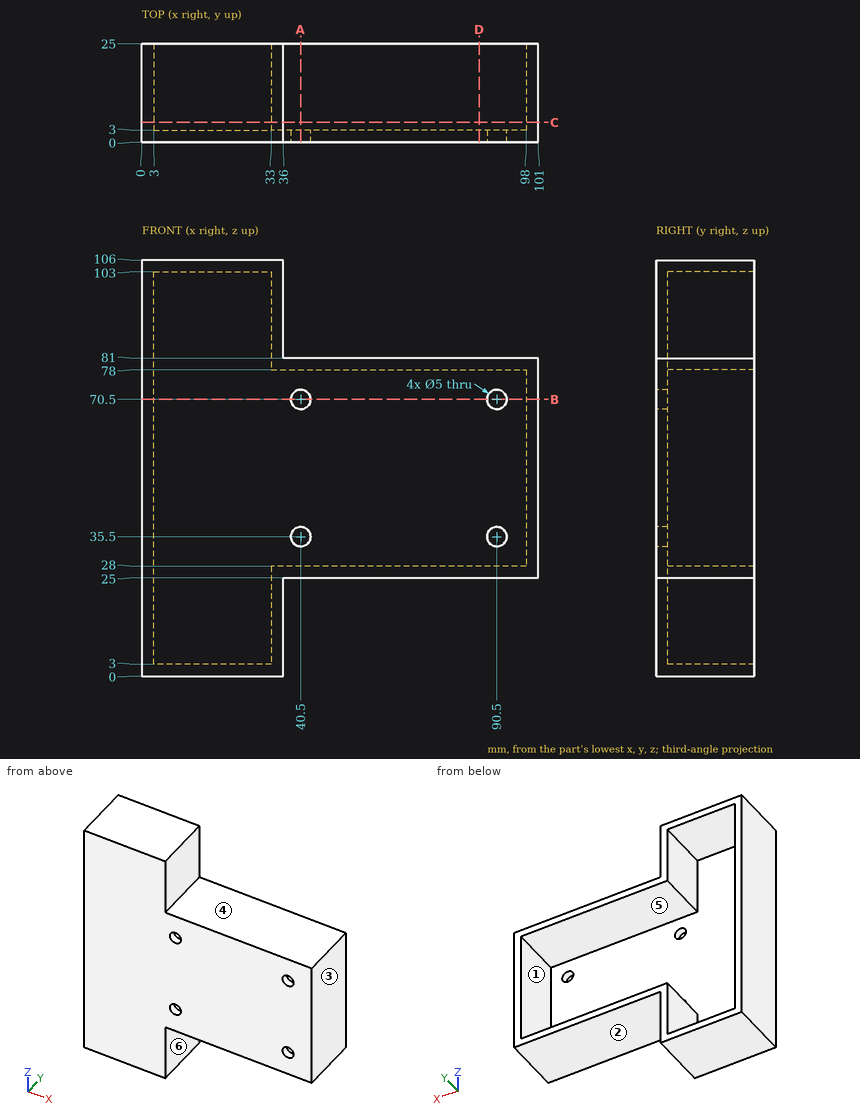
Part print with two shaded views. Sizes in mm from the minimum x, y, z corner. A direction names the side the tool comes from. Give positions to 0.01 mm unless a question says otherwise; leave off trailing zeros. Order: outer loops, then holes, each group sorted by start corner. A loop starts at its lowest first (then second) coordinate and runs counter-clockwise, first axis right, second up.
1) Saw through at C-C, the plane y = 5. Write the cut outline in (x, z), then the cut area to 3 significant figures.
2) Mould opens along Z. For the marked faces 1, 2 and 3 say: +Z half, -Z half, draft (parallel to the pull), parting line (faces both ways), or undercut.
3) Wall check: probe 1 along Z at (x, y) = (40.5, 1.8); probe 2 along X at (y, z) = (1.7, 35.5); probe 3 along X at (y, z) = (10.75, 15.5). Give the ranges that are in metal, low to high.
4) Saw through at A-A, the plane x = 40.5. Write the cut outline in (y, z).
5) Saw through at D-D, the plane x = 86. Write the cut outline in (y, z).
6) Pin check, flat tips, straight feed: pin 1 (1 mm diameter, centred on x = 39.5, y = 7, fed in from -Z); pin 2 (12.5 mm diameter, centred on y = 11, z = 16, fed in from +X); pin 3 (10 mm diameter, centred on x = 11.5, z = 32, fed in from +Y); pin 4 (3 mm diameter, centred on x = 40.5, z = 35.5, fed in from -Y). Stop position of each tip, or through.
7) 3-axis set-ups, long thin cutter, end or side, ignore diameter. For the marked faces 4, 5 and 6: which of +Z, -Z, +X, -X, +Y, -Y reach the whole face in a straight line?
8) Saw through at B-B, the plane z = 70.5. Write the cut outline in (x, y), then the cut area to 3 significant figures.
Computed:
1. outline: (0, 0) - (36, 0) - (36, 25) - (101, 25) - (101, 81) - (36, 81) - (36, 106) - (0, 106) - close; hole (3, 3) - (33, 3) - (33, 28) - (98, 28) - (98, 78) - (33, 78) - (33, 103) - (3, 103) - close
1. area: 1,210 mm2
2. face 1: undercut
2. face 2: -Z half
2. face 3: draft
3. probe 1: z = 25 to 33, 38 to 68, 73 to 81
3. probe 2: x = 0 to 38, 43 to 88, 93 to 101
3. probe 3: x = 0 to 3, 33 to 36
4. outline: (0, 25) - (25, 25) - (25, 28) - (3, 28) - (3, 33) - (0, 33) - close; (0, 38) - (3, 38) - (3, 68) - (0, 68) - close; (0, 73) - (3, 73) - (3, 78) - (25, 78) - (25, 81) - (0, 81) - close
5. outline: (0, 25) - (25, 25) - (25, 28) - (3, 28) - (3, 78) - (25, 78) - (25, 81) - (0, 81) - close
6. pin 1: stops at z = 25
6. pin 2: stops at x = 36
6. pin 3: stops at y = 3
6. pin 4: passes through
7. face 4: +Z, +X, +Y, -Y
7. face 5: +Y
7. face 6: -Z, +X, +Y, -Y
8. outline: (0, 0) - (38, 0) - (38, 3) - (3, 3) - (3, 25) - (0, 25) - close; (43, 0) - (88, 0) - (88, 3) - (43, 3) - close; (93, 0) - (101, 0) - (101, 25) - (98, 25) - (98, 3) - (93, 3) - close
8. area: 405 mm2
